Input: part model. Units: mm. Frame: model coordinates. Face numbers are marked on the shaded views. Round coordinates to 2 decimals unless told otherwise and drop trailing zeros. Loops run counter-clockwise (first coordinate to the right, second up) from the corner with the lowest first, then second, coordinate; pieces in that order, holes last. Notation, with made-up numbers: (-39, 63.25) -> (-13, 63.25) arc R30 cw to (-13, 87.25) -> close; hole circle Ø2 at (75.5, 47). An arc over 180 degrees is marked (long way). Answer in a Markdown table with one row per item. Add a question column.
Q1. Ray query, L1, parallel to Y at x = 0, z = 7.5; L2, parallel to Y at x = 0, z = -8; L3, parallel to Z at x = 7, y = -4. Return the intervals inside material, ascending. Write a range as from..to.
Q2. Section D-D, the plane z = 18. Output: boundary loops of the cut face in (x, y), and give its area (3 significant figures).
Q3. Pin query (flat end, axial travel): pin 1 (5 mm diameter, centred on x = -1.5, y = 1, fed in from +Z); pin 2 (1 mm diameter, centred on y = 4.5, z = 4, fed in from -X); pin 3 (1.5 mm diameter, centred on x = 1.5, z = -1, fed in from -Y). Return the tip coordinate at first contact, or that it passes through.
Q4. Section C-C, the plane y = 10.75. Output: boundary loops of the cut face in (x, z), and give its area (3 significant figures).
Q5. Section A-A, the plane z = -15.5. Output: boundary loops of the cut face in (x, y).
Q6. Section B-B, the plane y = -7. Output: boundary loops of the cut face in (x, z), and give its area (3 significant figures).
Q7. Mould query, pull axis Y, two halves, no side actions, for the marked faces 1, 2 and 3. Classes: pulls with the +Y half, pulls with the -Y half, needs draft (parallel to the pull), parting line crosses it, or undercut.
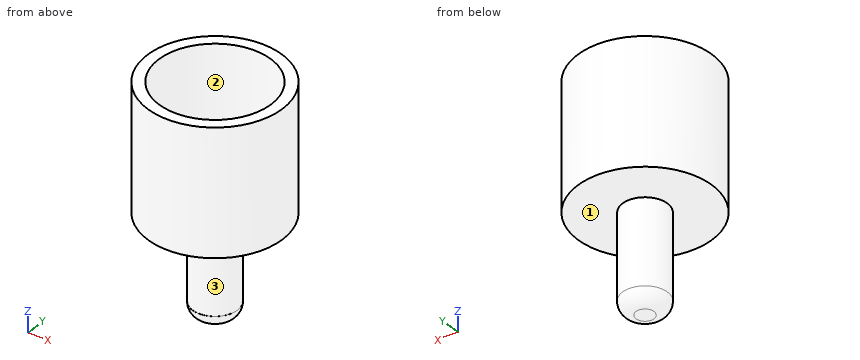
```python
from build123d import *

# Parameters (mm, degrees)
F0_R     = 15
F0_R_2   = 12.5
F7_DEPTH = 25
F0_R_3   = 5
F1_DEPTH = 3
F0_R_4   = 3.25
F2_DEPTH = 22
F3_R     = 5.0189857481
F4_DEPTH = 3
F5_R     = 2.99999
F6_R     = 2


# Not quite as in the source:
# - a fillet or chamfer is up to 0.001 mm smaller than in the source, because OpenCascade refuses the exact size


with BuildPart() as f7:
    # F0 (on Top) → F7 (new body)
    with BuildSketch(Plane.XY):
        Circle(F0_R)
        Circle(F0_R_2, mode=Mode.SUBTRACT)
    extrude(amount=F7_DEPTH)

    # F0 (on Top) → F1 (join)
    with BuildSketch(Plane.XY):
        Circle(F0_R)
        Circle(F0_R_2, mode=Mode.SUBTRACT)
        Circle(F0_R_2)
        Circle(F0_R_3, mode=Mode.SUBTRACT)
    extrude(amount=-F1_DEPTH)

    # F0 (on Top) → F2 (join)
    with BuildSketch(Plane.XY):
        Circle(F0_R_3)
        Circle(F0_R_4, mode=Mode.SUBTRACT)
    extrude(amount=-F2_DEPTH)

    # F3 (on face) → F4 (join)
    with BuildSketch(Plane(origin=(0, 0, -22), x_dir=(1, 0, 0), z_dir=(0, 0, -1))):
        Circle(F3_R)
    extrude(amount=F4_DEPTH)

    # F5 (radius 3 in the source; OpenCascade refuses exactly that, so slightly less here)
    f5_edges = [f7.edges().sort_by_distance(p)[0] for p in [
        (-5.018986, 0, -25),
    ]]
    fillet(f5_edges, radius=F5_R)

    # F6
    f6_edges = [f7.edges().sort_by_distance(p)[0] for p in [
        (-3.25, 0, 0),
    ]]
    fillet(f6_edges, radius=F6_R)


solid = f7.part
```
Answer block:
| question | item | result |
|---|---|---|
| 1 | L1 | -15..-12.5, 12.5..15 |
| 1 | L2 | -5..-3.25, 3.25..5 |
| 1 | L3 | -3..0 |
| 2 | outline | circle Ø30 at (0, 0); hole circle Ø25 at (0, 0) |
| 2 | area | 216 mm^2 |
| 3 | pin 1 | z = -0.24 |
| 3 | pin 2 | x = -14.46 |
| 3 | pin 3 | y = -14.98 |
| 4 | outline | (-10.46, -3) -> (10.46, -3) -> (10.46, 25) -> (6.38, 25) -> (6.38, 0) -> (-6.38, 0) -> (-6.38, 25) -> (-10.46, 25) -> close |
| 4 | area | 267 mm^2 |
| 5 | outline | circle Ø10 at (0, 0); hole circle Ø6.5 at (0, 0) |
| 6 | outline | (-13.27, -3) -> (13.27, -3) -> (13.27, 25) -> (10.36, 25) -> (10.36, 0) -> (-10.36, 0) -> (-10.36, 25) -> (-13.27, 25) -> close |
| 6 | area | 225 mm^2 |
| 7 | face 1 | needs draft |
| 7 | face 2 | undercut |
| 7 | face 3 | parting line crosses it |
